Here's how the part is built. I have some questions about the finished solid (model axes, mm). A direction names the side the tool comes from. Round coordinates to 2 decimals unless told otherwise and drop trailing zeros. Loops run counter-clockwise (first coordinate to the right, second up) from the corner with the lowest first, then second, coordinate; pieces in that order, holes last. Notation, with made-up numbers: (-10, 82) - (35, 82) arc R11 ccw to (35, 95) - close; hole circle Ø6 at (-10.75, -3). An arc over 180 degrees is marked (long way). Answer as a JSON object with one key per item and string values. Group by question number.
1) Which directions (+Z, -Z, +X, -X, +Y, -Y) give clear straight access to the entire face, cutting with the end or side of a thin tool? Please do faces 1 (the face through (-10.926, -3.441, -22.605)), 2 (the face through (0, -7, -8)).
2) Will these pins go through, and if not, where does the flat tip stop? P1, Ø5, axis at y = 4, z = -13.5, coming from the +X side; P2, Ø2, axis at x = 6, z = -9.5, coming from the +Y side; P3, Ø6, axis at x = 6, z = -15, coming from the -Y side.
3) I want a section at A-A, the plane y = 0. Please give me the cut outline in (x, z) (3 decimals), then the cut area to 3 significant figures.
4) I want a section at D-D, the plane z = -24.25. Please give me the cut outline in (x, y) (3 decimals).
5) If I drill on line 1 along Y through (x, z) = (0, -3.25) (3 decimals); line 2 along Y through (x, z) = (0, -9.75) (3 decimals); line 3 along Y through (x, z) = (1.5, -4.25), over which ranges is the centre line in solid material (lowest first)? Write a range as [from, to].
6) I want a section at C-C, the plane z = -12.75. Please give me the cut outline in (x, y) (3 decimals).
7) I want a section at B-B, the plane x = -2. Please give me the cut outline in (y, z).
from build123d import *

# Parameters (mm, degrees)
SKETCH1_3_R        = 1.190625
CUT_EXTRUDE1_DEPTH = 8
SKETCH1_R          = 2.8956
CUT_EXTRUDE2_DEPTH = 16


with BuildPart() as part:
    # Sketch2 → Revolve1 (revolve)
    with BuildSketch(Plane.YZ, mode=Mode.PRIVATE) as revolve1_sk:
        Polygon((0, 0), (9.525, 0), (9.525, -15), (11.455, -15), (11.455, -30), (0, -30), align=None)
    revolve(revolve1_sk.sketch.rotate(Axis((0, 0, -30), (0, 0, 1)), 90), axis=Axis((0, 0, -30), (0, 0, 1)))

    # Sketch1_3 → Cut-Extrude1 (cut)
    with BuildSketch(Plane(origin=(0, 0, 0), x_dir=(0, 1, 0), z_dir=(0, 0, 1))):
        with Locations(Location((0, 7.5, 0), (0, 0, 270))):
            Circle(SKETCH1_3_R)
        with Locations(Location((-7.5, 0, 0), (0, 0, 270))):
            Circle(SKETCH1_3_R)
        with Locations(Location((7.5, 0, 0), (0, 0, 270))):
            Circle(SKETCH1_3_R)
        with Locations(Location((0, -7.5, 0), (0, 0, 270))):
            Circle(SKETCH1_3_R)
    extrude(amount=-CUT_EXTRUDE1_DEPTH, mode=Mode.SUBTRACT)

    # Sketch1 → Cut-Extrude2 (cut)
    with BuildSketch(Plane(origin=(0, 0, 0), x_dir=(0, 1, 0), z_dir=(0, 0, 1))):
        with Locations(Location((0, 0, 0), (0, 0, 270))):
            Circle(SKETCH1_R)
    extrude(amount=-CUT_EXTRUDE2_DEPTH, mode=Mode.SUBTRACT)


solid = part.part
Outcome:
{
 "1": {"face 1": "+Z, -Z", "face 2": "+Z"},
 "2": {"P1": "x = 11.28", "P2": "y = 8.11", "P3": "y = -11.06"},
 "3": {"outline": "(-11.455, -30) - (11.455, -30) - (11.455, -15) - (9.525, -15) - (9.525, 0) - (8.691, 0) - (8.691, -8) - (6.309, -8) - (6.309, 0) - (2.896, 0) - (2.896, -16) - (-2.896, -16) - (-2.896, 0) - (-6.309, 0) - (-6.309, -8) - (-8.691, -8) - (-8.691, 0) - (-9.525, 0) - (-9.525, -15) - (-11.455, -15) - close", "area": "499 mm^2"},
 "4": {"outline": "circle Ø22.91 at (0, 0)"},
 "5": {"line 1": "[-9.525, -8.691], [-6.309, -2.896], [2.896, 6.309], [8.691, 9.525]", "line 2": "[-9.525, -2.896], [2.896, 9.525]", "line 3": "[-9.41, -2.48], [2.48, 9.41]"},
 "6": {"outline": "circle Ø19.05 at (0, 0); hole circle Ø5.791 at (0, 0)"},
 "7": {"outline": "(-11.28, -30) - (11.28, -30) - (11.28, -15) - (9.31, -15) - (9.31, 0) - (2.09, 0) - (2.09, -16) - (-2.09, -16) - (-2.09, 0) - (-9.31, 0) - (-9.31, -15) - (-11.28, -15) - close"}
}
